Input: part model. Units: mm. Frame: model coordinates. Round coordinates to 2 decimals unless told otherwise and drop trailing zeros. Write each loop counter-clockwise with the first axis right and the second up, starting at its lowest first coordinate (ties: lowest second). Pieces come first, ordered by that corner, then holes. Notation, with made-up numbers: M 85,30 L 133,30 A16 ccw 133,57 Z; hole C 60.25,-9.75 d6. An arc over 180 degrees is marked long. Answer as CSV lines item,"result". Start each with the question number.
```python
from build123d import *

# Parameters (mm, degrees)
SKETCH1_W           = 110
SKETCH1_H           = 139
BOSS_EXTRUDE1_DEPTH = 4
FILLET1_R           = 10


with BuildPart() as part:
    # Sketch1 → Boss-Extrude1 (new body)
    with BuildSketch(Plane(origin=(0, 0, 0), x_dir=(1, 0, 0), z_dir=(0, 1, 0))):
        Rectangle(SKETCH1_W, SKETCH1_H)
        with BuildLine():
            Line((-40.5, 58.5), (-37.5, 58.5))
            ThreePointArc((-37.5, 58.5), (-32, 53), (-37.5, 47.5))
            Line((-37.5, 47.5), (-40.5, 47.5))
            ThreePointArc((-40.5, 47.5), (-46, 53), (-40.5, 58.5))
        make_face(mode=Mode.SUBTRACT)
        with BuildLine():
            Line((37.5, 58.5), (40.5, 58.5))
            ThreePointArc((40.5, 58.5), (46, 53), (40.5, 47.5))
            Line((40.5, 47.5), (37.5, 47.5))
            ThreePointArc((37.5, 47.5), (32, 53), (37.5, 58.5))
        make_face(mode=Mode.SUBTRACT)
        with BuildLine():
            Line((-40.5, -47.5), (-37.5, -47.5))
            ThreePointArc((-37.5, -47.5), (-32, -53), (-37.5, -58.5))
            Line((-37.5, -58.5), (-40.5, -58.5))
            ThreePointArc((-40.5, -58.5), (-46, -53), (-40.5, -47.5))
        make_face(mode=Mode.SUBTRACT)
        with BuildLine():
            Line((37.5, -47.5), (40.5, -47.5))
            ThreePointArc((40.5, -47.5), (46, -53), (40.5, -58.5))
            Line((40.5, -58.5), (37.5, -58.5))
            ThreePointArc((37.5, -58.5), (32, -53), (37.5, -47.5))
        make_face(mode=Mode.SUBTRACT)
    extrude(amount=BOSS_EXTRUDE1_DEPTH)

    # Fillet1
    fillet1_edges = [part.edges().sort_by_distance(p)[0] for p in [
        (55, 2, 69.5),
        (-55, 2, 69.5),
        (-55, 2, -69.5),
        (55, 2, -69.5),
    ]]
    fillet(fillet1_edges, radius=FILLET1_R)


solid = part.part
```
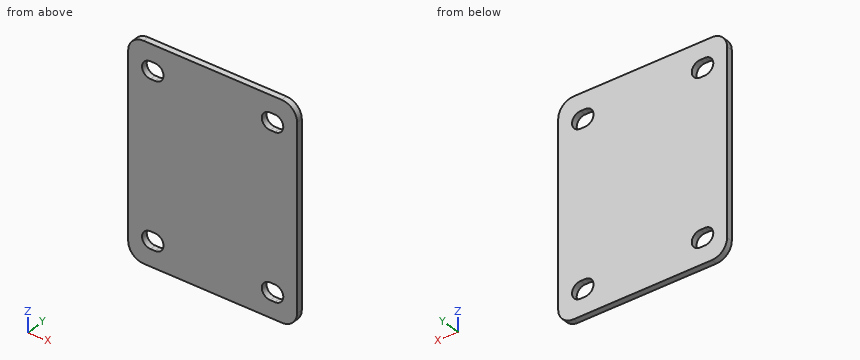
Item 1: Pin query (flat end, axial travel): pin 1 Ø2 at (x, z) = (-30.5, -32) entering from -Y. Return the tip coordinate at first contact, or that it passes through.
Item 2: Cut plane A-A, the plane y = 0.85. Return loops of the section in (x, z), plus the area to 3 significant figures.
Item 3: Cut plane B-B, the plane z = -53. Return loops of the section in (x, y), plus the area to 3 significant figures.
Item 4: Line query: line 1 (X direction, y = 1.9, z = 54.5); line 2 (X direction, y = 2.35, z = 48); line 3 (Z direction, x = 43.5, y = 3.1). Output: solid intervals per line, ascending. Write a range as [from, to].
Results list:
1,pin 1,"y = 0"
2,outline,"M -55,-59.5 A10 ccw -45,-69.5 L 45,-69.5 A10 ccw 55,-59.5 L 55,59.5 A10 ccw 45,69.5 L -45,69.5 A10 ccw -55,59.5 Z; hole M -40.5,-58.5 L -37.5,-58.5 A5.5 ccw -37.5,-47.5 L -40.5,-47.5 A5.5 ccw Z; hole M -40.5,47.5 L -37.5,47.5 A5.5 ccw -37.5,58.5 L -40.5,58.5 A5.5 ccw Z; hole M 37.5,-58.5 L 40.5,-58.5 A5.5 ccw 40.5,-47.5 L 37.5,-47.5 A5.5 ccw Z; hole M 37.5,47.5 L 40.5,47.5 A5.5 ccw 40.5,58.5 L 37.5,58.5 A5.5 ccw Z"
2,area,"14,700 mm²"
3,outline,"M -55,0 L -46,0 L -46,4 L -55,4 Z; M -32,0 L 32,0 L 32,4 L -32,4 Z; M 46,0 L 55,0 L 55,4 L 46,4 Z"
3,area,"328 mm²"
4,line 1,"[-55, -45.79], [-32.21, 32.21], [45.79, 55]"
4,line 2,"[-55, -42.79], [-35.21, 35.21], [42.79, 55]"
4,line 3,"[-69.5, -57.61], [-48.39, 48.39], [57.61, 69.5]"
